Build history of the part. All positions in model axes, mm. Coordinates: 2 decimals unless noted, no trailing zeros. Order: outer loops, then holes, each group sorted by start corner. A loop starts at its lowest first (then second) coordinate and runs counter-clockwise, first axis right, second up. Notation, with made-up numbers: (-8.75, 68.25) - (50.25, 68.25) arc R27 ccw to (50.25, 86.25) - close; hole circle Ø7 at (53.5, -7.5). An arc over 180 degrees is marked (long way). One line per item, written item: value.
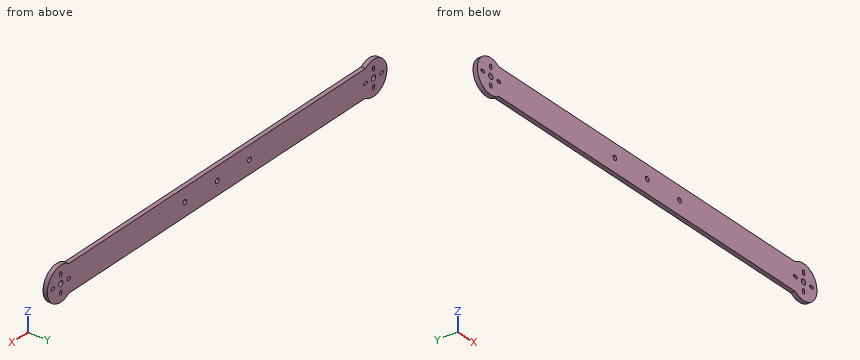
from build123d import *

# Parameters (mm, degrees)
BOSS_EXTRUDE1_DEPTH = 4
SKETCH2_R           = 2.5
CUT_EXTRUDE1_DEPTH  = 201.6938371
SKETCH3_R           = 2.159
CUT_EXTRUDE2_DEPTH  = 201.6938371


with BuildPart() as part:
    # Sketch1 → Boss-Extrude1 (new body)
    with BuildSketch(Plane(origin=(0, 0, 0), x_dir=(1, 0, 0), z_dir=(0, 1, 0))):
        with BuildLine():
            Line((-174.625, 12.7), (174.625, 12.7))
            ThreePointArc((174.625, 12.7), (200.025, 0), (174.625, -12.7))
            Line((174.625, -12.7), (-174.625, -12.7))
            ThreePointArc((-174.625, -12.7), (-200.025, 0), (-174.625, 12.7))
        make_face()
    extrude(amount=BOSS_EXTRUDE1_DEPTH)

    # Sketch2 → Cut-Extrude1 (cut, through all)
    with BuildSketch(Plane(origin=(0, 4, 0), x_dir=(1, 0, 0), z_dir=(0, 1, 0))):
        with Locations(Location((184.15, 0, 0), (0, 0, 270))):
            Circle(SKETCH2_R)
        with Locations(Location((-184.15, 0, 0), (0, 0, 90))):
            Circle(SKETCH2_R)
        with BuildLine():
            Line((173.691383345, 1.25), (175.608616655, 1.25))
            ThreePointArc((175.608616655, 1.25), (176.858616655, 0), (175.608616655, -1.25))
            Line((175.608616655, -1.25), (173.691383345, -1.25))
            ThreePointArc((173.691383345, -1.25), (172.441383345, 0), (173.691383345, 1.25))
        make_face()
        with BuildLine():
            Line((194.608616655, 1.25), (192.691383345, 1.25))
            ThreePointArc((192.691383345, 1.25), (191.441383345, 0), (192.691383345, -1.25))
            Line((192.691383345, -1.25), (194.608616655, -1.25))
            ThreePointArc((194.608616655, -1.25), (195.858616655, 0), (194.608616655, 1.25))
        make_face()
        with BuildLine():
            Line((185.4, 8.920928665), (185.4, 6.921035691))
            ThreePointArc((185.4, 6.921035691), (184.15, 5.671035691), (182.9, 6.921035691))
            Line((182.9, 6.921035691), (182.9, 8.920928665))
            ThreePointArc((182.9, 8.920928665), (184.15, 10.170928665), (185.4, 8.920928665))
        make_face()
        with BuildLine():
            Line((185.441381345, -9.078964309), (185.441381345, -7.078964309))
            ThreePointArc((185.441381345, -7.078964309), (184.191381345, -5.828964309), (182.941381345, -7.078964309))
            Line((182.941381345, -7.078964309), (182.941381345, -9.078964309))
            ThreePointArc((182.941381345, -9.078964309), (184.191381345, -10.328964309), (185.441381345, -9.078964309))
        make_face()
        with BuildLine():
            Line((-185.441381345, -9.078964309), (-185.441381345, -7.078964309))
            ThreePointArc((-185.441381345, -7.078964309), (-184.191381345, -5.828964309), (-182.941381345, -7.078964309))
            Line((-182.941381345, -7.078964309), (-182.941381345, -9.078964309))
            ThreePointArc((-182.941381345, -9.078964309), (-184.191381345, -10.328964309), (-185.441381345, -9.078964309))
        make_face()
        with BuildLine():
            Line((-185.4, 8.920928665), (-185.4, 6.921035691))
            ThreePointArc((-185.4, 6.921035691), (-184.15, 5.671035691), (-182.9, 6.921035691))
            Line((-182.9, 6.921035691), (-182.9, 8.920928665))
            ThreePointArc((-182.9, 8.920928665), (-184.15, 10.170928665), (-185.4, 8.920928665))
        make_face()
        with BuildLine():
            Line((-194.608616655, 1.25), (-192.691383345, 1.25))
            ThreePointArc((-192.691383345, 1.25), (-191.441383345, 0), (-192.691383345, -1.25))
            Line((-192.691383345, -1.25), (-194.608616655, -1.25))
            ThreePointArc((-194.608616655, -1.25), (-195.858616655, 0), (-194.608616655, 1.25))
        make_face()
        with BuildLine():
            Line((-173.691383345, 1.25), (-175.608616655, 1.25))
            ThreePointArc((-175.608616655, 1.25), (-176.858616655, 0), (-175.608616655, -1.25))
            Line((-175.608616655, -1.25), (-173.691383345, -1.25))
            ThreePointArc((-173.691383345, -1.25), (-172.441383345, 0), (-173.691383345, 1.25))
        make_face()
    extrude(amount=-CUT_EXTRUDE1_DEPTH, mode=Mode.SUBTRACT)

    # Sketch3 → Cut-Extrude2 (cut, through all)
    with BuildSketch(Plane(origin=(0, 4, 0), x_dir=(1, 0, 0), z_dir=(0, 1, 0))):
        with Locations(Location((0, 0, 0), (0, 0, 270))):
            Circle(SKETCH3_R)
        with Locations(Location((38.1, 0, 0), (0, 0, 270))):
            Circle(SKETCH3_R)
        with Locations(Location((-38.1, 0, 0), (0, 0, 270))):
            Circle(SKETCH3_R)
    extrude(amount=-CUT_EXTRUDE2_DEPTH, mode=Mode.SUBTRACT)


solid = part.part
1. Band-saw the part on B-B, the plane y = 2.2. Count the separate pieces of the cut face and the enclosed holes in it, and give its area (3 significant figures).
Values found:
separate pieces: 1
enclosed holes: 13
area: 10,100 mm2
2. Band-saw the part on A-A, the plane x = 30. Give the cut face in (y, z).
Values found:
outline: (0, -12.7) - (4, -12.7) - (4, 12.7) - (0, 12.7) - close
3. Probe line 1 along Z through (x, y) = (-184.15, 1.75) (3 decimals); line 2 along X through (y, z) = (2.7, 9); line 3 along X through (y, z) = (2.15, 1.5). List the from-to ranges inside material, lowest first.
Values found:
line 1: z = -15.875 to -10.171, -5.671 to -2.5, 2.5 to 5.83, 10.328 to 15.875
line 2: x = -197.23 to -185.44, -182.94 to 182.94, 185.44 to 197.23
line 3: x = -199.95 to -186.15, -182.15 to -39.65, -36.55 to -1.55, 1.55 to 36.55, 39.65 to 182.15, 186.15 to 199.95
4. Flat gauge pins, fed straight in: P1, Ø0.6, axis at x = 174.5, y = 2.5, coming from the -Z side; P2, Ø1.5, axis at x = -174.5, y = 2.5, coming from the -Z side; P3, Ø1, axis at y = 2.5, z = 8.5, coming from the -X side. Where does each tip first touch, or does it go through?
Values found:
P1: stops at z = -12.83
P2: stops at z = -13.15
P3: stops at x = -197.86
